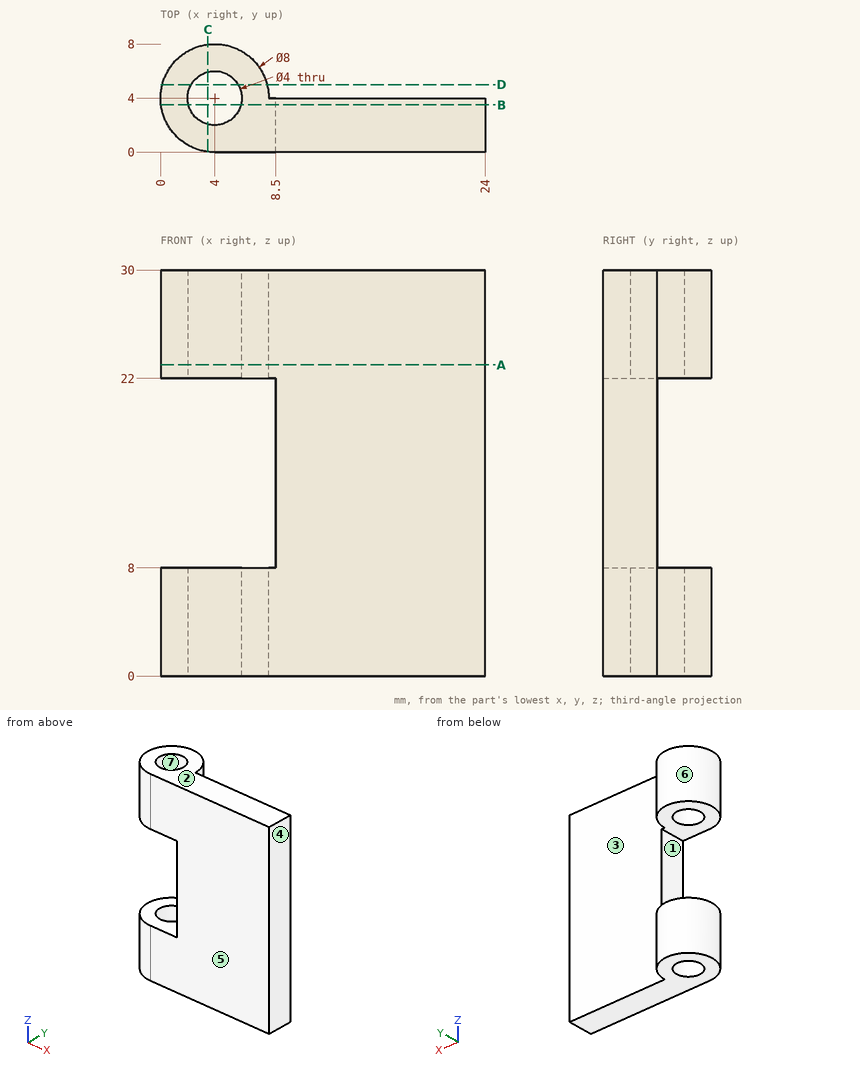
Print and shaded views of the part. All mm, measured from the part's lowest x, y and z. A direction names the side the tool comes from. Round coordinates to 2 decimals unless told otherwise and drop trailing zeros. Write each loop counter-clockwise with the first axis right and the second up, starting at its lowest first coordinate (ties: lowest second). Pieces come first, ordered by that corner, then holes. Notation, with made-up numbers: (13, 1) -> (70, 1) arc R29 cw to (70, 31) -> close; hole circle Ø5 at (80.5, -28.75). An arc over 180 degrees is marked (long way). Write item = value, one per line.
(1) Flat gauge pins, fed straight in: pin 1 (4.5 mm diameter, centred on y = 1, z = 13.5, fed in from -X); pin 2 (5 mm diameter, centred on x = 18, z = 19, fed in from +Y). Where does each tip first touch, or does it go through?
Answer:
pin_1 = 8.5
pin_2 = 4
(2) Probe L1, parallel to Z at x = 4.5, y = 6.25; L2, parallel to X at y = 2.5, z = 21.75; L3, parallel to Y at x = 2.25, z = 4. List the from-to ranges inside material, lowest first.
Answer:
L1 = 0 to 8, 22 to 30
L2 = 8.5 to 24
L3 = 0.4 to 3.03, 4.97 to 7.6
(3) Band-saw the part on D-D (y = 5). Give the cut face in (x, z).
Answer:
outline = (0.13, 0) -> (2.27, 0) -> (2.27, 8) -> (0.13, 8) -> close; (0.13, 22) -> (2.27, 22) -> (2.27, 30) -> (0.13, 30) -> close; (5.73, 0) -> (7.87, 0) -> (7.87, 8) -> (5.73, 8) -> close; (5.73, 22) -> (7.87, 22) -> (7.87, 30) -> (5.73, 30) -> close
(4) Band-saw the part on B-B (y = 3.5). Give the cut face in (x, z), then the cut area to 3 significant figures.
Answer:
outline = (0.03, 0) -> (2.06, 0) -> (2.06, 8) -> (0.03, 8) -> close; (0.03, 22) -> (2.06, 22) -> (2.06, 30) -> (0.03, 30) -> close; (5.94, 0) -> (24, 0) -> (24, 30) -> (5.94, 30) -> (5.94, 22) -> (8.5, 22) -> (8.5, 8) -> (5.94, 8) -> close
area = 539 mm2
(5) Band-saw the part on C-C (x = 3.5). Give the cut face in (y, z).
Answer:
outline = (0.03, 0) -> (2.06, 0) -> (2.06, 8) -> (0.03, 8) -> close; (0.03, 22) -> (2.06, 22) -> (2.06, 30) -> (0.03, 30) -> close; (5.94, 0) -> (7.97, 0) -> (7.97, 8) -> (5.94, 8) -> close; (5.94, 22) -> (7.97, 22) -> (7.97, 30) -> (5.94, 30) -> close
(6) Band-saw the part on A-A (z = 23). Give the cut face in (x, y), then the cut area to 3 significant figures.
Answer:
outline = (4, 0) -> (24, 0) -> (24, 4) -> (8, 4) arc R4 ccw (long way) to start; hole circle Ø4 at (4, 4)
area = 105 mm2
(7) Two-plate mould, pull along X, no slides. Class the marked faces 4, 5, 6 and 7: pulls with the +X half, pulls with the -X half, needs draft (parallel to the pull), parting line crosses it, or undercut.
Answer:
face_4 = pulls with the +X half
face_5 = needs draft
face_6 = parting line crosses it
face_7 = undercut
(8) Tool access for the marked faces 1, 2 and 3: list every direction of +Z, -Z, +X, -X, +Y, -Y with a clear straight run to the whole face (end or side of a thin tool).
Answer:
face_1 = -X, +Y, -Y
face_2 = +Z, +X, -X, +Y, -Y
face_3 = +Z, -Z, +X, +Y
